Read the model definition and answer for the solid it produces. Units are mm, in the model's axes. A direction names the side the tool comes from. Coordinates: 2 decimals unless noted, no trailing zeros. Order: outer loops, then holes, each group sorted by start corner. A loop starts at its lowest first (then second) coordinate and runs counter-clockwise, first axis right, second up. Notation, with made-up numbers: M -28,16 L 19,16 A26 ccw 19,52 Z; hole C 53,23.25 d5. An arc over 180 degrees is marked long. One line per question, with ' | ' between items. Start each with the question number.
1) The mould has two halves that part along Z. Classify faces 6 (the face through (15.517, 24, -4)), 7 (the face through (1, 0, -4)), 8 (the face through (-18.193, 27, -4)), 9 (the face through (32.029, 27.542, 22.572)): +Z half, -Z half, draft (parallel to the pull), parting line (faces both ways), or undercut.
2) Find section C-C, the plane y = 41. Write down the section's boundary in (x, z), plus the area to 3 significant figures.
3) Find section D-D, the plane x = 17. Write down the section's boundary in (y, z).
4) A tool of negligible diameter and unlimited length cuts with its end or side. For faces 1 (the face through (18.64, 53.08, -4.45)), 2 (the face through (-0.75, -19.41, -8.88)), 3 (the face through (20.089, 32, -4)), 4 (the face through (-16.67, 53.16, -4.45)), 5 (the face through (18, 24, -21.447)), from which of +Z, -Z, +X, -X, +Y, -Y can it reach the whole face along a straight path? Write none if from no direction.
5) Consider probe 1 along Y at (x, z) = (-4, -11.5); probe 2 along Z at (x, y) = (23.5, 39); probe 3 along Y at (x, z) = (15, -15.5). Determine where each line is inside the solid, lowest interval first.
6) Find section B-B, the plane z = 3. Write down the section's boundary in (x, y).
7) Find section A-A, the plane x = 0. Write down the section's boundary in (y, z), plus the area to 3 significant figures.
8) Given P1, Ø8.5, axis at x = 3.5, z = -4.5, coming from the +Y side; P2, Ø8, axis at x = 12.5, z = -3.5, coming from the -Y side; P3, Ø3.5, axis at x = 18.5, z = 2.5, coming from the -Y side, each flat-ended and moving along its own axis, determine where each tip first touches the part or whether it passes through.
from build123d import *

# Parameters (mm, degrees)
F0_W         = 38.2822398096
F0_H         = 52.1388202906
F1_DEPTH     = 54.61
F2_R         = 5.728059517
F3_DEPTH     = 39.37
F4_W         = 6.2229996547
F4_H         = 34.6710011363
F5_DEPTH     = 4.572
F6_R         = 4.1653363511
F7_DEPTH     = 18.796
F8_W         = 67.563995719
F8_H         = 76.8984956667
F9_DEPTH     = 2.286
F10_T1_DEPTH = 64.8388202906
F10_T3_DEPTH = 88.7771779414
F10_T5_DEPTH = 98.1116778891


# Not quite as in the source:
# - a fillet or chamfer that OpenCascade refuses, or shapes differently, is made with other operations: its cross-section is extruded or revolved along the edge and cut away or added


with BuildPart() as f1:
    # F0 (on Front) → F1 (new body)
    with BuildSketch(Plane.XZ):
        with Locations((0.9477725253, -4.0886364877)):
            Rectangle(F0_W, F0_H)
    extrude(amount=-F1_DEPTH)

    # F2 (on Front) → F3 (join)
    with BuildSketch(Plane.XZ):
        with Locations((0, -14.5573755726)):
            Circle(F2_R)
    extrude(amount=F3_DEPTH)

    # F4 (on face) → F5 (cut)
    with BuildSketch(Plane.YZ.offset(20.0888924301)):
        with Locations((11.2236249261, -4.1116252542)):
            Rectangle(F4_W, F4_H)
        with Locations((24.1141221486, -4.1116252542)):
            Rectangle(F4_W, F4_H)
    extrude(amount=-F5_DEPTH, mode=Mode.SUBTRACT)

    # F6 (on face) → F7 (join)
    with BuildSketch(Plane(origin=(0, 54.61, 0), x_dir=(-1, 0, 0), z_dir=(0, 1, 0))):
        with Locations((0, 9.3980003148)):
            Circle(F6_R)
    extrude(amount=F7_DEPTH)

    # F8 (on face) → F9 (join)
    with BuildSketch(Plane.XY.offset(21.9807736576)):
        with Locations((0.1111254096, 27.0033725537)):
            Rectangle(F8_W, F8_H)
    extrude(amount=F9_DEPTH)

    # F10: fillet of radius 5.08 on 8 edges, made by hand

    # F10_s2 → F10_t1 (cut)
    with BuildSketch(Plane.XY.offset(-42.858046633)):
        with BuildLine():
            ThreePointArc((20.0888924301, 5.08), (18.6009948785, 1.4878975516), (15.0088924301, 0))
            Line((15.0088924301, 0), (20.0888924301, 0))
            Line((20.0888924301, 0), (20.0888924301, 5.08))
        make_face()
        with BuildLine():
            ThreePointArc((-18.1933473796, 5.08), (-16.705449828, 1.4878975516), (-13.1133473796, 0))
            Line((-13.1133473796, 0), (-18.1933473796, 0))
            Line((-18.1933473796, 0), (-18.1933473796, 5.08))
        make_face()
        with BuildLine():
            ThreePointArc((-13.1133473796, 54.61), (-16.705449828, 53.1221024484), (-18.1933473796, 49.53))
            Line((-18.1933473796, 49.53), (-18.1933473796, 54.61))
            Line((-18.1933473796, 54.61), (-13.1133473796, 54.61))
        make_face()
        with BuildLine():
            ThreePointArc((20.0888924301, 49.53), (18.6009948785, 53.1221024484), (15.0088924301, 54.61))
            Line((15.0088924301, 54.61), (20.0888924301, 54.61))
            Line((20.0888924301, 54.61), (20.0888924301, 49.53))
        make_face()
    extrude(amount=F10_T1_DEPTH, mode=Mode.SUBTRACT)

    # F10_s4 → F10_t3 (cut)
    with BuildSketch(Plane.YZ.offset(-44.2774635611)):
        with BuildLine():
            ThreePointArc((65.4526203871, 24.2667736576), (63.6196395196, 22.5886421747), (61.2099839426, 21.9807736576))
            Line((61.2099839426, 21.9807736576), (65.4526203871, 21.9807736576))
            Line((65.4526203871, 21.9807736576), (65.4526203871, 24.2667736576))
        make_face()
        with BuildLine():
            ThreePointArc((-11.4458752796, 24.2667736576), (-9.6128944122, 22.5886421747), (-7.2032388351, 21.9807736576))
            Line((-7.2032388351, 21.9807736576), (-11.4458752796, 21.9807736576))
            Line((-11.4458752796, 21.9807736576), (-11.4458752796, 24.2667736576))
        make_face()
    extrude(amount=F10_T3_DEPTH, mode=Mode.SUBTRACT)

    # F10_s6 → F10_t5 (cut)
    with BuildSketch(Plane.XZ.offset(-76.0592114983)):
        with BuildLine():
            ThreePointArc((29.6504868246, 21.9807736576), (32.0601424016, 22.5886421747), (33.8931232691, 24.2667736576))
            Line((33.8931232691, 24.2667736576), (33.8931232691, 21.9807736576))
            Line((33.8931232691, 21.9807736576), (29.6504868246, 21.9807736576))
        make_face()
        with BuildLine():
            ThreePointArc((-33.6708724499, 24.2667736576), (-31.8378915824, 22.5886421747), (-29.4282360054, 21.9807736576))
            Line((-29.4282360054, 21.9807736576), (-33.6708724499, 21.9807736576))
            Line((-33.6708724499, 21.9807736576), (-33.6708724499, 24.2667736576))
        make_face()
    extrude(amount=F10_T5_DEPTH, mode=Mode.SUBTRACT)


solid = f1.part
Report:
1) face 6: undercut | face 7: undercut | face 8: draft | face 9: -Z half
2) outline: M -33.67,24.27 A5.08 ccw -29.43,21.98 L -18.19,21.98 L -18.19,-30.16 L 20.09,-30.16 L 20.09,21.98 L 29.65,21.98 A5.08 ccw 33.89,24.27 Z | area: 2,140 mm^2
3) outline: M -11.45,24.27 A5.08 ccw -7.2,21.98 L 0.41,21.98 L 0.41,-30.16 L 54.2,-30.16 L 54.2,21.98 L 61.21,21.98 A5.08 ccw 65.45,24.27 Z; hole M 8.11,-21.45 L 14.34,-21.45 L 14.34,13.22 L 8.11,13.22 Z; hole M 21,-21.45 L 27.23,-21.45 L 27.23,13.22 L 21,13.22 Z
4) face 1: -Z, +X, +Y | face 2: -Y | face 3: -Z, +X, +Y, -Y | face 4: -Z, -X, +Y | face 5: +X
5) probe 1: y = -39.37 to 54.61 | probe 2: z = 21.98 to 24.27 | probe 3: y = 0 to 54.61
6) outline: M -18.19,5.08 A5.08 ccw -13.11,0 L 15.01,0 A5.08 ccw 20.09,5.08 L 20.09,8.11 L 15.52,8.11 L 15.52,14.34 L 20.09,14.34 L 20.09,21 L 15.52,21 L 15.52,27.23 L 20.09,27.23 L 20.09,49.53 A5.08 ccw 15.01,54.61 L -13.11,54.61 A5.08 ccw -18.19,49.53 Z
7) outline: M -39.37,-20.29 L 0,-20.29 L 0,-30.16 L 54.61,-30.16 L 54.61,5.23 L 73.41,5.23 L 73.41,13.56 L 54.61,13.56 L 54.61,21.98 L 61.21,21.98 A5.08 ccw 65.45,24.27 L -11.45,24.27 A5.08 ccw -7.2,21.98 L 0,21.98 L 0,-8.83 L -39.37,-8.83 Z | area: 3,620 mm^2
8) P1: stops at y = 54.61 | P2: stops at y = 0 | P3: stops at y = 0.31
